The listing builds one solid part. Answer for the finished solid, in the listing's coordinates (mm). A direction names the side the tool comes from. Coordinates: 2 decimals unless noted, no trailing zeros. Loops run counter-clockwise (first coordinate to the right, second up) from the corner with the lowest first, then second, coordinate; pieces in that order, holes last. Notation, with made-up numbers: (78, 77) - (91, 77) arc R10 cw to (91, 88) - close; hole circle Ø7 at (-8.5, -26). An arc over 180 degrees is marked (long way). Write each question's results on one line, items separated by ' | '. Start each with the question number.
(1) Find section B-B on x = -3.5. Determine the outline of the cut face in (y, z).
(2) For faces 5 (the flat face through (-26, 50, 114)), 6 (the flat face through (-22, 62, 20)), 7 (the flat face through (23.05, 50, 121)), determine the directions among +Z, -Z, +X, -X, +Y, -Y from which every point of the face is accessible in a straight line to the end or side of a thin tool.
(3) Find section C-C on z = 39. Determine the outline of the cut face in (x, y).
(4) Determine the mould class of faces 1 (the flat face through (27, 50, 20)), 2 (the flat face through (-20.595, 58, 10)), 3 (the flat face through (-23.05, 50, 121)), 4 (the flat face through (24.05, 57, 10)) for opening direction X: released by +X, released by -X, zero draft, split by the parting line, or undercut.
(5) Consider line 1 (Y direction, x = 21.5, z = 40); line 2 (X direction, y = 69.5, z = 16); line 3 (Z direction, x = -22, y = 56.5). Determine where each line is inside the solid, lowest interval first. Write a range as from..to.
(6) Given pin 1 Ø2.5 at (x, y) = (27, 50) entering from -Z; pin 2 Ø6.5 at (y, z) = (55, 14.5) entering from -X; pin 3 Ø8 at (x, y) = (-22.5, 65) entering from +Z; pin 4 Ø5 at (y, z) = (55.5, 82.5) entering from +X, each flat-ended and moving along its own axis, determine where each tip first touches the part or whether it passes through.
(7) Find section A-A on y = 54.25. Determine the outline of the cut face in (x, z).
from build123d import *

# Parameters (mm, degrees)
BOSS_EXTRUDE1_DEPTH = 20
SKETCH2_W           = 5
SKETCH2_H           = 3
BOSS_EXTRUDE2_DEPTH = 120
SKETCH4_W           = 6
SKETCH4_H           = 14
CUT_EXTRUDE1_DEPTH  = 10


with BuildPart() as part:
    # Sketch1 → Boss-Extrude1 (new body)
    with BuildSketch(Plane.XY):
        with BuildLine():
            Line((-24.05, 64.8), (-24.05, 48.8))
            Line((-24.05, 48.8), (24.05, 48.8))
            Line((24.05, 48.8), (24.05, 64.8))
            add(Edge.make_bspline(
                [(24.05, 64.8), (22.187774265, 77.400108054), (20.594686421, 64.8)],
                knots=[0, 0, 0, 1, 1, 1], degree=2))
            Line((20.594686421, 64.8), (20.594686421, 51.8))
            Line((20.594686421, 51.8), (-20.594686421, 51.8))
            Line((-20.594686421, 51.8), (-20.594686421, 64.8))
            add(Edge.make_bspline(
                [(-24.05, 64.8), (-22.187774265, 77.400108054), (-20.594686421, 64.8)],
                knots=[0, 0, 0, 1, 1, 1], degree=2))
        make_face()
    extrude(amount=BOSS_EXTRUDE1_DEPTH)

    # Sketch2 → Boss-Extrude2 (add)
    with BuildSketch(Plane.XY.offset(20)):
        with Locations((-26.55, 50.3)):
            Rectangle(SKETCH2_W, SKETCH2_H)
        Polygon((-24.05, 51.8), (-24.05, 48.8), (24.05, 48.8), (24.05, 51.8), (20.594686421, 51.8), (-20.594686421, 51.8), align=None)
        with Locations((26.55, 50.3)):
            Rectangle(SKETCH2_W, SKETCH2_H)
    extrude(amount=BOSS_EXTRUDE2_DEPTH)

    # Sketch4 → Cut-Extrude1 (cut)
    with BuildSketch(Plane(origin=(0, 51.8, 0), x_dir=(1, 0, 0), z_dir=(0, 1, 0))):
        with Locations((-26.05, -121)):
            Rectangle(SKETCH4_W, SKETCH4_H)
        with Locations((26.05, -121)):
            Rectangle(SKETCH4_W, SKETCH4_H)
    extrude(amount=-CUT_EXTRUDE1_DEPTH, mode=Mode.SUBTRACT)


solid = part.part
Values:
1) outline: (48.8, 0) - (51.8, 0) - (51.8, 140) - (48.8, 140) - close
2) face 5: -X, +Y, -Y | face 6: +Z, +X, -X, +Y | face 7: +X, +Y, -Y
3) outline: (-29.05, 48.8) - (29.05, 48.8) - (29.05, 51.8) - (-29.05, 51.8) - close
4) face 1: zero draft | face 2: undercut | face 3: released by -X | face 4: released by +X
5) line 1: y = 48.8..51.8 | line 2: x = -23.14..-21.4, 21.4..23.14 | line 3: z = 0..20
6) pin 1: stops at z = 20 | pin 2: stops at x = -24.05 | pin 3: stops at z = 20 | pin 4: passes through
7) outline: (-24.05, 0) - (-20.59, 0) - (-20.59, 20) - (-24.05, 20) - close; (20.59, 0) - (24.05, 0) - (24.05, 20) - (20.59, 20) - close
